Source: CAD feature listing. Evaluate the final solid. Frame: model axes, mm. Give positions to 0.01 mm unless a question says otherwise; leave off trailing zeros. Write each loop counter-clockwise with the first axis right and the second up, starting at its lowest first coordinate (ties: lowest second). Pieces come first, ordered by that corner, then holes. Notation, with made-up numbers: (44, 67) -> (86, 67) arc R15 cw to (86, 77) -> close; hole circle Ø8 at (9.5, -29.5). An arc over 180 degrees is marked (long way). Answer as a JSON object with one key per item and string values. Group by question number.
Item 1: First-contact query: pin 1 Ø1.5 at (x, y) = (-12, 2.5) entering from +Z; pin 2 Ø6 at (x, z) = (4.5, 16) entering from +Y; pin 3 Ø1.5 at (y, z) = (3, 13.5) entering from -X; pin 4 Ø2.5 at (y, z) = (2.5, 4.5) entering from -X. Flat tips, straight axial feed; report the tip coordinate or a pass-through.
Item 2: Pull-direction query (X, two-part tool) for faces 1 (the face through (20, 0, 1)), 2 (the face through (60.65, 2.54, 14.51)), 3 (the face through (83.04, 2.46, -8.22)), 4 (the face through (46.17, 2.54, -5.54)); classes: pulls with the +X half, pulls with the -X half, needs draft (parallel to the pull), parting line crosses it, or undercut.
Item 3: Section query C-C on y = 2.15. Give the number of separate pieces and of enclosed holes in the cut face, plus the area to 3 significant figures.
Item 4: Section query A-A on x = 24. Return the cut outline in (y, z).
Item 5: Ray query, probe 1 along Z at (x, y) = (-3.5, 3.2); probe 2 along X at (y, z) = (3.7, -0.5); probe 3 along Z at (x, y) = (-29, 3.4). Return the intervals inside material, ascending. Write a range as from..to.
Item 6: Section query B-B on x = -83. Return the cut outline in (y, z).
Item 7: Section query D-D on x = 49. Return the cut outline in (y, z).
from build123d import *

# Parameters (mm, degrees)
SKETCH1_R           = 1.65
SKETCH1_R_2         = 3
BOSS_EXTRUDE1_DEPTH = 5
CUT_EXTRUDE1_DEPTH  = 5
SKETCH3_R           = 3
BOSS_EXTRUDE2_DEPTH = 5
FILLET1_R           = 10


with BuildPart() as part:
    # Sketch1 → Boss-Extrude1 (new body)
    with BuildSketch(Plane(origin=(0, 0, 0), x_dir=(1, 0, 0), z_dir=(0, 1, 0))):
        with BuildLine():
            Line((-75, 11.5), (75, 11.5))
            ThreePointArc((75, 11.5), (86.5, 0), (75, -11.5))
            Line((75, -11.5), (-75, -11.5))
            ThreePointArc((-75, -11.5), (-86.5, 0), (-75, 11.5))
        make_face()
        with Locations((-75, 8)):
            Circle(SKETCH1_R, mode=Mode.SUBTRACT)
        with Locations((-67, 0)):
            Circle(SKETCH1_R, mode=Mode.SUBTRACT)
        with Locations((-75, -8)):
            Circle(SKETCH1_R, mode=Mode.SUBTRACT)
        with Locations((-83, 0)):
            Circle(SKETCH1_R, mode=Mode.SUBTRACT)
        with Locations((75, 0)):
            Circle(SKETCH1_R_2, mode=Mode.SUBTRACT)
        with Locations((-75, 0)):
            Circle(SKETCH1_R_2, mode=Mode.SUBTRACT)
    extrude(amount=BOSS_EXTRUDE1_DEPTH)

    # Sketch2 → Cut-Extrude1 (cut)
    with BuildSketch(Plane(origin=(0, 5, 0), x_dir=(1, 0, 0), z_dir=(0, 1, 0))):
        with BuildLine():
            Line((-63.77502784, 2.5), (-46.452027549, 2.5))
            Line((-46.452027549, 2.5), (-67.254033308, 8.5))
            ThreePointArc((-67.254033308, 8.5), (-65.051425718, 5.768524054), (-63.77502784, 2.5))
        make_face()
        Polygon((-56.429022412, 8.5), (-35.627016654, 2.5), (-35.627016654, 8.5), align=None)
        Polygon((-12.325010896, 2.5), (-33.127016654, 8.5), (-33.127016654, 2.5), align=None)
        Polygon((-1.5, 8.5), (-22.302005758, 8.5), (-1.5, 2.5), align=None)
        Polygon((-1.5, -2.5), (-1.5, -8.5), (-22.302005758, -8.5), align=None)
        Polygon((-33.127016654, -2.5), (-12.325010896, -2.5), (-33.127016654, -8.5), align=None)
        Polygon((-35.627016654, -2.5), (-35.627016654, -8.5), (-56.429022412, -8.5), align=None)
        with BuildLine():
            Line((-46.452027549, -2.5), (-67.254033308, -8.5))
            ThreePointArc((-67.254033308, -8.5), (-65.051425718, -5.768524054), (-63.77502784, -2.5))
            Line((-63.77502784, -2.5), (-46.452027549, -2.5))
        make_face()
        Polygon((22.302005758, -8.5), (1.5, -2.5), (1.5, -8.5), align=None)
        Polygon((33.127016654, -8.5), (33.127016654, -2.5), (12.325010896, -2.5), align=None)
        Polygon((56.429022412, -8.5), (35.627016654, -2.5), (35.627016654, -8.5), align=None)
        with BuildLine():
            Line((46.452027549, -2.5), (67.254033308, -8.5))
            ThreePointArc((67.254033308, -8.5), (65.051425718, -5.768524054), (63.77502784, -2.5))
            Line((63.77502784, -2.5), (46.452027549, -2.5))
        make_face()
        with BuildLine():
            Line((46.452027549, 2.5), (67.254033308, 8.5))
            ThreePointArc((67.254033308, 8.5), (65.051425718, 5.768524054), (63.77502784, 2.5))
            Line((63.77502784, 2.5), (46.452027549, 2.5))
        make_face()
        Polygon((35.627016654, 2.5), (35.627016654, 8.5), (56.429022412, 8.5), align=None)
        Polygon((33.127016654, 2.5), (12.325010896, 2.5), (33.127016654, 8.5), align=None)
        Polygon((1.5, 2.5), (1.5, 8.5), (22.302005758, 8.5), align=None)
    extrude(amount=-CUT_EXTRUDE1_DEPTH, mode=Mode.SUBTRACT)

    # Sketch3 → Boss-Extrude2 (add, through all)
    with BuildSketch(Plane(origin=(0, 5, 0), x_dir=(1, 0, 0), z_dir=(0, 1, 0))):
        with BuildLine():
            Line((86.5, 0), (86.5, -28.5))
            ThreePointArc((86.5, -28.5), (75, -40), (63.5, -28.5))
            Line((63.5, -28.5), (63.5, 0))
            ThreePointArc((63.5, 0), (75, 11.5), (86.5, 0))
        make_face()
        with Locations((75, 0)):
            Circle(SKETCH3_R, mode=Mode.SUBTRACT)
    extrude(amount=-BOSS_EXTRUDE2_DEPTH)

    # Fillet1
    fillet1_edges = [part.edges().sort_by_distance(p)[0] for p in [
        (63.5, 2.5, 11.5),
    ]]
    fillet(fillet1_edges, radius=FILLET1_R)


solid = part.part
Worked answers:
{
 "1": {"pin 1": "z = 11.5", "pin 2": "through", "pin 3": "x = 58.34", "pin 4": "x = -86.03"},
 "2": {"face 1": "needs draft", "face 2": "pulls with the -X half", "face 3": "pulls with the +X half", "face 4": "undercut"},
 "3": {"separate pieces": "1", "enclosed holes": "22", "area": "3,480 mm^2"},
 "4": {"outline": "(0, -11.5) -> (5, -11.5) -> (5, -5.87) -> (0, -5.87) -> close; (0, -2.5) -> (5, -2.5) -> (5, 2.5) -> (0, 2.5) -> close; (0, 5.87) -> (5, 5.87) -> (5, 11.5) -> (0, 11.5) -> close"},
 "5": {"probe 1": "-11.5..-8.5, -3.08..3.08, 8.5..11.5", "probe 2": "-86.49..-84.57, -81.43..-77.96, -72.04..-68.57, -65.43..72.04, 77.96..86.49", "probe 3": "-11.5..-7.31, -2.5..2.5, 7.31..11.5"},
 "6": {"outline": "(0, -8.26) -> (5, -8.26) -> (5, -1.65) -> (0, -1.65) -> close; (0, 1.65) -> (5, 1.65) -> (5, 8.26) -> (0, 8.26) -> close"},
 "7": {"outline": "(0, -11.5) -> (5, -11.5) -> (5, -8.5) -> (0, -8.5) -> close; (0, -6.36) -> (5, -6.36) -> (5, -3.23) -> (0, -3.23) -> close; (0, -2.5) -> (5, -2.5) -> (5, 2.5) -> (0, 2.5) -> close; (0, 3.23) -> (5, 3.23) -> (5, 6.36) -> (0, 6.36) -> close; (0, 8.5) -> (5, 8.5) -> (5, 11.5) -> (0, 11.5) -> close"}
}
